Source: CAD feature listing. Evaluate the final solid. Frame: model axes, mm. A direction names the side the tool comes from. Round coordinates to 2 decimals unless told otherwise and drop trailing zeros. Order: outer loops, then holes, each group sorted by start corner. A loop starts at its lowest first (then second) coordinate and runs counter-clockwise, first axis right, second up. Notation, with made-up numbers: (12, 75) -> (69, 75) arc R38 ccw to (69, 114) -> close; hole circle Ø9 at (25, 44). An arc over 180 degrees is marked (long way). Write item = value, one per line. Start each with the question number.
(1) Cut plane B-B on y = 13.25. Return the cut outline in (x, z).
(2) Ray query, line 1 (X direction, y = 4.5, z = 2); line 2 (Z direction, x = 0, y = 13.75); line 3 (X direction, y = 20.5, z = 7). Return the intervals inside material, ascending.
(3) Reachability of faces 4 (the face through (0, 5, 1.5)), 5 (the face through (4, 0, 4)), 6 (the face through (4, 1, 7.8)), 7 (the face through (0, -1, 1.5)) from +Z, -Z, +X, -X, +Y, -Y: full face, straight path, thin tool, end or side. Return the list, or none.
(4) Cut plane A-A on z = 7. Return the cut outline in (x, y).
(5) Draft query along Z for faces 1 (the face through (4.18, 12.1, 8.7)), 2 (the face through (-2, 9.335, 7)), 3 (the face through (-0.04, 21.9, 0.57)). Return one class per face: released by +Z, released by -Z, zero draft, split by the parting line, or undercut.
(6) Contact query for flat-ended pins moving along their axis: pin 1 Ø0.8 at (x, z) = (-1.5, 8.5) entering from -Y; pin 2 Ø5 at (x, y) = (-3, 18) entering from -Z; pin 3 Ø0.8 at (x, y) = (-0.5, -1) entering from +Z; pin 4 Ø0.7 at (x, y) = (-4, 1) entering from +Z. Output: stop coordinate, or through.
(7) Cut plane D-D on z = 5. Return the cut outline in (x, y).
from build123d import *

# Parameters (mm, degrees)
F0_W         = 1.3692331631
F0_H         = 7.834737435
F0_W_2       = 6.5
F0_H_2       = 0.9
F0_W_3       = 0.6192331631
F0_H_3       = 1.05
F0_H_4       = 13.165262565
F0_W_4       = 0.8807668369
F0_W_5       = 1.6307668369
F1_DEPTH     = 0.9
F2_DEPTH     = 1.5
F3_DEPTH     = 7.8
F5_W         = 9.5
F5_H         = 19.2867757659
F6_DEPTH     = 1.5
F7_R         = 3
F8_DEPTH     = 22.501
F9_T1_DEPTH  = 5.3
F9_T3_DEPTH  = 5.5
F9_T5_DEPTH  = 22.2867757659
F9_T7_DEPTH  = 27
F9_S11_W     = 2
F9_S11_H     = 2
F9_T12_DEPTH = 2
F9_S17_W     = 2
F9_S17_H     = 2
F9_T18_DEPTH = 2
F9_S23_W     = 2
F9_S23_H     = 2
F9_T24_DEPTH = 2
F9_S29_W     = 2
F9_S29_H     = 2
F9_T30_DEPTH = 2


# Not quite as in the source:
# - a fillet or chamfer that OpenCascade refuses, or shapes differently, is made with other operations: its cross-section is extruded or revolved along the edge and cut away or added
# - a feature names something its author has since deleted; it is built from what else it names


with BuildPart() as f1:
    # F0 (on Top) → F1 (new body)
    with BuildSketch(Plane.XY):
        Polygon((-4.75, 1.5), (-4.75, -1.5), (-3.3807668369, -1.5), (-3.3807668369, -0.45), (-4, -0.45), (-4, 0.45), (-3.3807668369, 0.45), (-3.3807668369, 1.5), align=None)
        Polygon((-3.3807668369, -0.45), (-3.3807668369, -1.5), (-3.1192331631, -1.5), (3.1192331631, -1.5), (3.1192331631, -0.45), align=None)
        with Locations((-4.0653834185, 5.4173687175)):
            Rectangle(F0_W, F0_H)
        with Locations((-0.1307668369, 0)):
            Rectangle(F0_W_2, F0_H_2)
        with Locations((-3.6903834185, 0)):
            Rectangle(F0_W_3, F0_H_2)
        with Locations((-0.1307668369, 5.4173687175)):
            Rectangle(F0_W_2, F0_H)
        with Locations((-0.1307668369, 0.975)):
            Rectangle(F0_W_2, F0_H_3)
        with Locations((-4.0653834185, 15.9173687175)):
            Rectangle(F0_W, F0_H_4)
        Polygon((3.1192331631, -0.45), (3.1192331631, -1.5), (3.3807668369, -1.5), (4.75, -1.5), (4.75, 1.5), (3.1192331631, 1.5), (3.1192331631, 0.45), (4, 0.45), (4, -0.45), align=None)
        with Locations((3.5596165815, 0)):
            Rectangle(F0_W_4, F0_H_2)
        with Locations((3.9346165815, 5.4173687175)):
            Rectangle(F0_W_5, F0_H)
        with Locations((-0.1307668369, 15.9173687175)):
            Rectangle(F0_W_2, F0_H_4)
        with Locations((3.9346165815, 15.9173687175)):
            Rectangle(F0_W_5, F0_H_4)
    extrude(amount=F1_DEPTH)

    # F0 (on Top) → F2 (join)
    with BuildSketch(Plane.XY):
        Polygon((-3.3807668369, -0.45), (-3.3807668369, -1.5), (-3.1192331631, -1.5), (3.1192331631, -1.5), (3.1192331631, -0.45), align=None)
        Polygon((3.1192331631, -0.45), (3.1192331631, -1.5), (3.3807668369, -1.5), (4.75, -1.5), (4.75, 1.5), (3.1192331631, 1.5), (3.1192331631, 0.45), (4, 0.45), (4, -0.45), align=None)
        Polygon((-4.75, 1.5), (-4.75, -1.5), (-3.3807668369, -1.5), (-3.3807668369, -0.45), (-4, -0.45), (-4, 0.45), (-3.3807668369, 0.45), (-3.3807668369, 1.5), align=None)
        with Locations((-0.1307668369, 0.975)):
            Rectangle(F0_W_2, F0_H_3)
        with Locations((-4.0653834185, 5.4173687175)):
            Rectangle(F0_W, F0_H)
        with Locations((3.9346165815, 5.4173687175)):
            Rectangle(F0_W_5, F0_H)
        with Locations((-0.1307668369, 5.4173687175)):
            Rectangle(F0_W_2, F0_H)
        with Locations((-4.0653834185, 15.9173687175)):
            Rectangle(F0_W, F0_H_4)
        with Locations((-0.1307668369, 15.9173687175)):
            Rectangle(F0_W_2, F0_H_4)
        with Locations((3.9346165815, 15.9173687175)):
            Rectangle(F0_W_5, F0_H_4)
    extrude(amount=F2_DEPTH)

    # F0 (on Top) → F3 (join)
    with BuildSketch(Plane.XY):
        Polygon((-4.75, 1.5), (-4.75, -1.5), (-3.3807668369, -1.5), (-3.3807668369, -0.45), (-4, -0.45), (-4, 0.45), (-3.3807668369, 0.45), (-3.3807668369, 1.5), align=None)
        Polygon((3.1192331631, -0.45), (3.1192331631, -1.5), (3.3807668369, -1.5), (4.75, -1.5), (4.75, 1.5), (3.1192331631, 1.5), (3.1192331631, 0.45), (4, 0.45), (4, -0.45), align=None)
        with Locations((-4.0653834185, 5.4173687175)):
            Rectangle(F0_W, F0_H)
        with Locations((3.9346165815, 5.4173687175)):
            Rectangle(F0_W_5, F0_H)
        with Locations((-4.0653834185, 15.9173687175)):
            Rectangle(F0_W, F0_H_4)
        with Locations((-0.1307668369, 15.9173687175)):
            Rectangle(F0_W_2, F0_H_4)
        with Locations((3.9346165815, 15.9173687175)):
            Rectangle(F0_W_5, F0_H_4)
    extrude(amount=F3_DEPTH)

    # F5 (on offset) → F6 (join)
    with BuildSketch(Plane.XY.offset(7.8)):
        with Locations((0, 12.856612117)):
            Rectangle(F5_W, F5_H)
    extrude(amount=F6_DEPTH)

    # F7 (on Front) → F8 (cut, through all)
    with BuildSketch(Plane.XZ):
        with Locations((0, 4.5)):
            Circle(F7_R)
    extrude(amount=-F8_DEPTH, mode=Mode.SUBTRACT)

    # F9: fillet of radius 2 on 8 edges, made by hand

    # F9_s2 → F9_t1 (cut)
    with BuildSketch(Plane.XY.offset(2)):
        with BuildLine():
            ThreePointArc((4.75, 20.5), (4.1642135624, 21.9142135624), (2.75, 22.5))
            Line((2.75, 22.5), (4.75, 22.5))
            Line((4.75, 22.5), (4.75, 20.5))
        make_face()
        with BuildLine():
            ThreePointArc((-4.75, 20.5), (-4.1642135624, 21.9142135624), (-2.75, 22.5))
            Line((-2.75, 22.5), (-4.75, 22.5))
            Line((-4.75, 22.5), (-4.75, 20.5))
        make_face()
    extrude(amount=F9_T1_DEPTH, mode=Mode.SUBTRACT)

    # F9_s4 → F9_t3 (cut)
    with BuildSketch(Plane.YZ.offset(-2.75)):
        with BuildLine():
            ThreePointArc((20.5, 9.3), (21.9142135624, 8.7142135624), (22.5, 7.3))
            Line((22.5, 7.3), (22.5, 9.3))
            Line((22.5, 9.3), (20.5, 9.3))
        make_face()
        with BuildLine():
            ThreePointArc((20.5, 0), (21.9142135624, 0.5857864376), (22.5, 2))
            Line((22.5, 2), (22.5, 0))
            Line((22.5, 0), (20.5, 0))
        make_face()
    extrude(amount=F9_T3_DEPTH, mode=Mode.SUBTRACT)

    # F9_s6 → F9_t5 (cut)
    with BuildSketch(Plane.XZ.offset(-20.5)):
        with BuildLine():
            ThreePointArc((4.75, 7.3), (4.1642135624, 8.7142135624), (2.75, 9.3))
            Line((2.75, 9.3), (4.75, 9.3))
            Line((4.75, 9.3), (4.75, 7.3))
        make_face()
        with BuildLine():
            ThreePointArc((-4.75, 7.3), (-4.1642135624, 8.7142135624), (-2.75, 9.3))
            Line((-2.75, 9.3), (-4.75, 9.3))
            Line((-4.75, 9.3), (-4.75, 7.3))
        make_face()
    extrude(amount=F9_T5_DEPTH, mode=Mode.SUBTRACT)

    # F9_s8 → F9_t7 (cut)
    with BuildSketch(Plane.XZ.offset(-20.5)):
        with BuildLine():
            ThreePointArc((2.75, 0), (4.1642135624, 0.5857864376), (4.75, 2))
            Line((4.75, 2), (4.75, 0))
            Line((4.75, 0), (2.75, 0))
        make_face()
        with BuildLine():
            ThreePointArc((-4.75, 2), (-4.1642135624, 0.5857864376), (-2.75, 0))
            Line((-2.75, 0), (-4.75, 0))
            Line((-4.75, 0), (-4.75, 2))
        make_face()
    extrude(amount=F9_T7_DEPTH, mode=Mode.SUBTRACT)


with BuildPart() as f9_tool10:
    # F9_s11 → F9_t12 (new body)
    with BuildSketch(Plane.YZ.offset(2.75)):
        with Locations((21.5, 8.3)):
            Rectangle(F9_S11_W, F9_S11_H)
    extrude(amount=F9_T12_DEPTH)

    # F9_s13 → F9_t14 (revolve, cut)
    with BuildSketch(Plane(origin=(2.75, 20.5, 7.3), x_dir=(0, -0.7071067812, -0.7071067812), z_dir=(0, -0.7071067812, 0.7071067812))):
        with BuildLine():
            ThreePointArc((0, -2), (2, 0), (0, 2))
            Line((0, 2), (0, -2))
        make_face()
    revolve(axis=Axis((2.75, 20.5, 7.3), (1, 0, 0)), mode=Mode.SUBTRACT)


with BuildPart() as f1_1:
    add(f1.part)

    # F9_t9: cut F9_tool10
    add(f9_tool10.part, mode=Mode.SUBTRACT)


with BuildPart() as f9_tool16:
    # F9_s17 → F9_t18 (new body)
    with BuildSketch(Plane.XY.offset(2)):
        with Locations((3.75, 21.5)):
            Rectangle(F9_S17_W, F9_S17_H)
    extrude(amount=-F9_T18_DEPTH)

    # F9_s19 → F9_t20 (revolve, cut)
    with BuildSketch(Plane(origin=(2.75, 20.5, 2), x_dir=(-0.7071067812, -0.7071067812, 0), z_dir=(0.7071067812, -0.7071067812, 0))):
        with BuildLine():
            ThreePointArc((0, -2), (2, 0), (0, 2))
            Line((0, 2), (0, -2))
        make_face()
    revolve(axis=Axis((2.75, 20.5, 2), (0, 0, -1)), mode=Mode.SUBTRACT)


with BuildPart() as f1_2:
    add(f1_1.part)

    # F9_t15: cut F9_tool16
    add(f9_tool16.part, mode=Mode.SUBTRACT)


with BuildPart() as f9_tool22:
    # F9_s23 → F9_t24 (new body)
    with BuildSketch(Plane.YZ.offset(-2.75)):
        with Locations((21.5, 8.3)):
            Rectangle(F9_S23_W, F9_S23_H)
    extrude(amount=-F9_T24_DEPTH)

    # F9_s25 → F9_t26 (revolve, cut)
    with BuildSketch(Plane(origin=(-2.75, 20.5, 7.3), x_dir=(0, -0.7071067812, -0.7071067812), z_dir=(0, 0.7071067812, -0.7071067812))):
        with BuildLine():
            ThreePointArc((0, -2), (2, 0), (0, 2))
            Line((0, 2), (0, -2))
        make_face()
    revolve(axis=Axis((-2.75, 20.5, 7.3), (-1, 0, 0)), mode=Mode.SUBTRACT)


with BuildPart() as f1_3:
    add(f1_2.part)

    # F9_t21: cut F9_tool22
    add(f9_tool22.part, mode=Mode.SUBTRACT)


with BuildPart() as f9_tool28:
    # F9_s29 → F9_t30 (new body)
    with BuildSketch(Plane.YZ.offset(-2.75)):
        with Locations((21.5, 1)):
            Rectangle(F9_S29_W, F9_S29_H)
    extrude(amount=-F9_T30_DEPTH)

    # F9_s31 → F9_t32 (revolve, cut)
    with BuildSketch(Plane(origin=(-2.75, 20.5, 2), x_dir=(0, -0.7071067812, 0.7071067812), z_dir=(0, -0.7071067812, -0.7071067812))):
        with BuildLine():
            ThreePointArc((0, -2), (2, 0), (0, 2))
            Line((0, 2), (0, -2))
        make_face()
    revolve(axis=Axis((-2.75, 20.5, 2), (-1, 0, 0)), mode=Mode.SUBTRACT)


with BuildPart() as f1_4:
    add(f1_3.part)

    # F9_t27: cut F9_tool28
    add(f9_tool28.part, mode=Mode.SUBTRACT)


solid = f1_4.part
Evaluation:
q1.outline = (-4.75, 2) arc R2 ccw to (-2.75, 0) -> (2.75, 0) arc R2 ccw to (4.75, 2) -> (4.75, 7.3) arc R2 ccw to (2.75, 9.3) -> (-2.75, 9.3) arc R2 ccw to (-4.75, 7.3) -> close; hole circle Ø6 at (0, 4.5)
q2.line_1 = -4.75 to -3.38, 3.12 to 4.75
q2.line_2 = 0 to 1.5, 7.5 to 9.3
q2.line_3 = -4.75 to -1.66, 1.66 to 4.75
q3.face_4 = -Y
q3.face_5 = +Z
q3.face_6 = +Z, +X, -X, -Y
q3.face_7 = +Z, -Y
q4.outline = (-4.75, -1.5) -> (-3.38, -1.5) -> (-3.38, -0.45) -> (-4, -0.45) -> (-4, 0.45) -> (-3.38, 0.45) -> (-3.38, 9.33) -> (-1.66, 9.33) -> (-1.66, 22.5) -> (-2.75, 22.5) arc R2 ccw to (-4.75, 20.5) -> close; (1.66, 9.33) -> (3.12, 9.33) -> (3.12, 0.45) -> (4, 0.45) -> (4, -0.45) -> (3.12, -0.45) -> (3.12, -1.5) -> (4.75, -1.5) -> (4.75, 20.5) arc R2 ccw to (2.75, 22.5) -> (1.66, 22.5) -> close
q5.face_1 = released by +Z
q5.face_2 = undercut
q5.face_3 = released by -Z
q6.pin_1 = 3.21
q6.pin_2 = 0
q6.pin_3 = 1.5
q6.pin_4 = 7.8
q7.outline = (-4.75, -1.5) -> (-3.38, -1.5) -> (-3.38, -0.45) -> (-4, -0.45) -> (-4, 0.45) -> (-3.38, 0.45) -> (-3.38, 9.33) -> (-2.96, 9.33) -> (-2.96, 22.49) arc R2 ccw to (-4.75, 20.5) -> close; (2.96, 9.33) -> (3.12, 9.33) -> (3.12, 0.45) -> (4, 0.45) -> (4, -0.45) -> (3.12, -0.45) -> (3.12, -1.5) -> (4.75, -1.5) -> (4.75, 20.5) arc R2 ccw to (2.96, 22.49) -> close
